Geometry: final body of the model. Coordinates: model frame, mm. Round coordinates to 2 decimals unless told otherwise and drop trailing zeros. Order: outer loops, then holes, each group sorted by start corner. A loop starts at its lowest first (then second) coordinate and runs counter-clockwise, first axis right, second up. Notation, with made-up numbers: (64, 31.25) - (82, 31.25) arc R11 cw to (82, 41.25) - close; hole circle Ø4 at (8, -3). An arc over 180 degrees is marked (long way). Put each result on its own line as item: value. Start each with the question number.
(1) Material intervals for L1, parallel to Y at x = 48.5, z = -144.5; L2, parallel to Y at x = 626, z = -76, sorted ascending. Write a range as [from, to].
(2) Section A-A (x = 122). Output: boundary loops of the cut face in (y, z), and give its area (3 significant figures).
(3) Section C-C (z = 175.5). Output: boundary loops of the cut face in (x, y), and give its area (3 significant figures).
(4) Section B-B (y = 142.5). Output: boundary loops of the cut face in (x, z), and give its area (3 significant figures).
(5) Pin query (flat end, axial travel): P1, Ø8, axis at x = 558, z = -117.5, coming from the +Y side; P2, Ø3, axis at x = 240, z = 70, coming from the +Y side; P3, Ø3, axis at x = 446, z = 174, coming from the +Y side. Return the tip coordinate at first contact, or that it passes through.
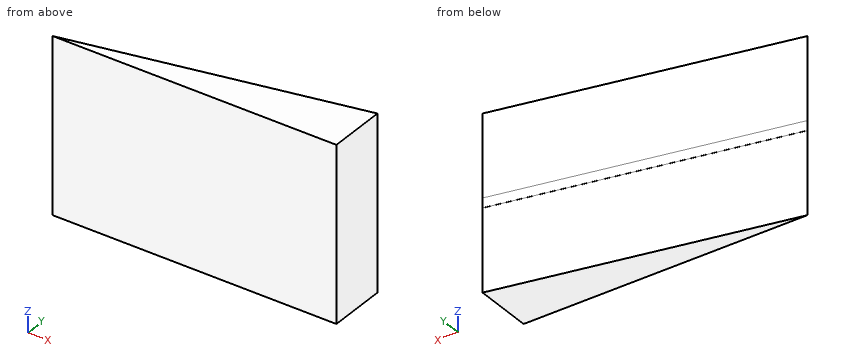
Autodesk Inventor part; units mm, degrees
ref_plane "YZ Plane" through (0, 0, 0) normal (1, 0, 0) x (0, 1, 0)
ref_plane "XZ Plane" through (0, 0, 0) normal (0, 1, 0) x (-1, 0, 0)
ref_plane "XY Plane" through (0, 0, 0) normal (0, 0, 1) x (1, 0, 0)
sketch "Sketch1" plane through (0, 0, 0) normal (0, 0, 1) x (1, 0, 0)
  line L0 (0, 0) -> (746.6045, 152.4)
  line L1 (0, 182.88) -> (0, -30.48)
  line L2 (-149.3209, 0) -> (895.9254, 0)
  line L3 (746.6045, 152.4) -> (746.6045, 0)
  line L4 (0, 0) -> (746.6045, 0)
  dimension "d0" = 152.4
  dimension "d1" = 762
extrude "Extrusion1" add sketch "Sketch1" along normal mid plane 457.2
sketch "Sketch4" plane through (0, 0, 228.6) normal (-0.2, 0.9798, 0) x (0.9798, 0.2, 0)
  line L0 (914.4, 228.6) -> (-152.4, 228.6)
  line L1 (762, 215.9) -> (0, 215.9)
  line L2 (0, 215.9) -> (0, 241.3)
  line L3 (0, 241.3) -> (762, 241.3)
  line L4 (762, 241.3) -> (762, 215.9)
  line L5 (762, 215.9) -> (0, 241.3) construction
  line L6 (0, 215.9) -> (762, 241.3) construction
  line L7 (0, 0) -> (0, 457.2)
  line L8 (762, 0) -> (0, 0)
  line L9 (762, 457.2) -> (762, 0)
  line L10 (0, 457.2) -> (762, 457.2)
  line L11 (762, 457.2) -> (762, 0)
  line L12 (0, 0) -> (0, 457.2)
  point P0 (0, 228.6)
  point P1 (381, 228.6)
  dimension "d6" = 25.4
extrude "Extrusion2" add sketch "Sketch4" along normal blind 0.254 contours L4 L1 L2 L0 | L0 L2 L3 L4
properties part number "Ramp"
Checks:
1. L1: y = [0, 9.9]
1. L2: y = [0, 127.78]
2. outline: (0, -228.6) - (24.9, -228.6) - (24.9, -12.7) - (25.16, -12.7) - (25.16, 12.7) - (24.9, 12.7) - (24.9, 228.6) - (0, 228.6) - close
2. area: 11,400 mm²
3. outline: (0, 0) - (746.6, 0) - (746.6, 152.4) - close
3. area: 56,900 mm²
4. outline: (696.84, -12.7) - (698.1, -12.7) - (698.1, -228.6) - (746.6, -228.6) - (746.6, 228.6) - (698.1, 228.6) - (698.1, 12.7) - (696.84, 12.7) - close
4. area: 22,200 mm²
5. P1: stops at y = 114.72
5. P2: stops at y = 49.3
5. P3: stops at y = 91.35
